from build123d import *

# Parameters (mm, degrees)
SKETCH1_R             = 57.5
BOSS_EXTRUDE1_DEPTH   = 27
SKETCH2_R             = 7.5
CUT_EXTRUDE1_DEPTH    = 86.68255365
SKETCH3_R             = 2.0950865
CUT_EXTRUDE2_DEPTH    = 21.472569
CIRPATTERN1_START     = 5.527430651
CIRPATTERN1_OUTLINE_R = 2.0950865
CIRPATTERN1_DEPTH     = 21.472569349


# Read off the part's stored shape, not the designer's step: CirPattern1
with BuildPart() as part:
    # Sketch1 → Boss-Extrude1 (new body)
    with BuildSketch(Plane(origin=(0, 0, 0), x_dir=(1, 0, 0), z_dir=(0, 1, 0))):
        with Locations(Location((0, 0, 0), (0, 0, 270))):
            Circle(SKETCH1_R)
    extrude(amount=BOSS_EXTRUDE1_DEPTH)

    # Sketch2 → Cut-Extrude1 (cut, through all)
    with BuildSketch(Plane(origin=(0, 0, 0), x_dir=(1, 0, 0), z_dir=(0, 1, 0))):
        with Locations(Location((0, 0, 0), (0, 0, 270))):
            Circle(SKETCH2_R)
    extrude(amount=CUT_EXTRUDE1_DEPTH, mode=Mode.SUBTRACT)

    # Sketch3 → Cut-Extrude2 (cut)
    with BuildSketch(Plane(origin=(0, 27, 0), x_dir=(1, 0, 0), z_dir=(0, 1, 0))):
        with Locations(Location((-24.087177083, 0, 0), (0, 0, 270))):
            Circle(SKETCH3_R)
    extrude(amount=-CUT_EXTRUDE2_DEPTH, mode=Mode.SUBTRACT)

    # CirPattern1 outline → CirPattern1 (cut)
    with BuildSketch(Plane(origin=(0, 0, 0), x_dir=(1, 0, 0), z_dir=(0, 1, 0)).offset(CIRPATTERN1_START)):
        with Locations((-17.032206255, -17.032206255)):
            Circle(CIRPATTERN1_OUTLINE_R)
        with Locations((-17.032206255, 17.032206255)):
            Circle(CIRPATTERN1_OUTLINE_R)
        with Locations((0, 24.087177083)):
            Circle(CIRPATTERN1_OUTLINE_R)
        with Locations((17.032206255, 17.032206255)):
            Circle(CIRPATTERN1_OUTLINE_R)
        with Locations((24.087177083, 0)):
            Circle(CIRPATTERN1_OUTLINE_R)
        with Locations((17.032206255, -17.032206255)):
            Circle(CIRPATTERN1_OUTLINE_R)
        with Locations((0, -24.087177083)):
            Circle(CIRPATTERN1_OUTLINE_R)
    extrude(amount=CIRPATTERN1_DEPTH, mode=Mode.SUBTRACT)


solid = part.part
Model file for the job. Use its own axes, mm. A direction names the side the tool comes from. Coordinates: 2 decimals unless noted, no trailing zeros. Write each loop counter-clockwise with the first axis right and the second up, starting at its lowest first coordinate (ties: lowest second). Pieces come first, ordered by that corner, then holes. Notation, with made-up numbers: (6, 17.25) -> (26, 17.25) arc R21 cw to (26, 46.25) -> close; hole circle Ø11 at (76.25, 47.25). An arc over 180 degrees is marked (long way). One line per item, written item: value. Start each with the question number.
1) Probe probe 1 along X at (y, z) = (6.75, -5); probe 2 along X at (y, z) = (16.75, -25); probe 3 along X at (y, z) = (13.5, -16). List the from-to ranges inside material, lowest first.
2) Which spindle directions (+Z, -Z, +X, -X, +Y, -Y) get a long thin tool onto all of the face, cutting with end or side? Do faces 1 (the face through (0, 5.527, -24)), 2 (the face through (1, 27, 12)). Say none if no direction does.
3) Slice it at D-D on z = -13. Write the cut outline in (x, y).
4) Slice it at B-B on z = 0. Write the cut outline in (x, y).
5) Slice it at C-C on y = 7. Count the separate pieces of the cut face and the enclosed holes in it, then the cut area to 3 significant figures.
6) Slice it at A-A on x = 0. Write the cut outline in (y, z), then the cut area to 3 significant figures.
7) Pull direction Z, two halves, no side cores. Call faces 3 (the face through (1, 0, 12)), 4 (the face through (17, 5.527, 17)), 5 (the face through (0.33, 13.311, -7.493)): +Z half, -Z half, draft (parallel to the pull), parting line (faces both ways), or undercut.
8) Flat gauge pins, fed straight in: pin 1 Ø6 at (x, y) = (27, 17.5) entering from -Z; pin 2 Ø1.3 at (x, z) = (24, 1) entering from +Y; pin 3 Ø6 at (x, y) = (19.5, 24) entering from +Z; pin 4 Ø12 at (x, z) = (0, 0) entering from +Y. Where does each tip first touch, or does it go through?
Answers follow:
1. probe 1: -57.28 to -5.59, 5.59 to 57.28
1. probe 2: -51.78 to -1.89, 1.89 to 51.78
1. probe 3: -55.23 to -18.86, -15.21 to 15.21, 18.86 to 55.23
2. face 1: +Y
2. face 2: +Z, -Z, +X, -X, +Y
3. outline: (-56.01, 0) -> (56.01, 0) -> (56.01, 27) -> (-56.01, 27) -> close
4. outline: (-57.5, 0) -> (-7.5, 0) -> (-7.5, 27) -> (-21.99, 27) -> (-21.99, 5.53) -> (-26.18, 5.53) -> (-26.18, 27) -> (-57.5, 27) -> close; (7.5, 0) -> (57.5, 0) -> (57.5, 27) -> (26.18, 27) -> (26.18, 5.53) -> (21.99, 5.53) -> (21.99, 27) -> (7.5, 27) -> close
5. separate pieces: 1
5. enclosed holes: 9
5. area: 10,100 mm2
6. outline: (0, -57.5) -> (27, -57.5) -> (27, -26.18) -> (5.53, -26.18) -> (5.53, -21.99) -> (27, -21.99) -> (27, -7.5) -> (0, -7.5) -> close; (0, 7.5) -> (27, 7.5) -> (27, 21.99) -> (5.53, 21.99) -> (5.53, 26.18) -> (27, 26.18) -> (27, 57.5) -> (0, 57.5) -> close
6. area: 2,520 mm2
7. face 3: draft
7. face 4: undercut
7. face 5: undercut
8. pin 1: z = -52.25
8. pin 2: y = 5.53
8. pin 3: z = 55.08
8. pin 4: through
